Work out the finished part from the listing and answer in its coordinate system (mm). A direction names the side the tool comes from. Coordinates: 2 decimals unless noted, no trailing zeros. Order: outer loops, then holes, each group sorted by start corner. A loop starts at its lowest first (then second) coordinate and runs counter-clockwise, first axis right, second up. Notation, with made-up numbers: M 36.25,84 L 86.25,84 A29 cw 86.25,110 Z; hole C 24.25,37.25 d3. An arc over 180 degrees is marked long. Use a Markdown table: item, result.
from build123d import *

# Parameters (mm, degrees)
ESQUISSE1_R                  = 76.2
ESQUISSE1_R_2                = 60
BOSS_EXTRU_1_DEPTH           = 10
ESQUISSE2_W                  = 30
ESQUISSE2_H                  = 3
BOSS_EXTRU_2_DEPTH           = 480
R_P_TITION_CIRCULAIRE1_COUNT = 4
R_P_TITION_LIN_AIRE1_COUNT   = 2
R_P_TITION_LIN_AIRE1_PITCH   = 490
ESQUISSE5_R                  = 76.2
ESQUISSE5_R_2                = 62.5
BOSS_EXTRU_3_DEPTH           = 10
R_P_TITION_LIN_AIRE2_COUNT   = 2
R_P_TITION_LIN_AIRE2_PITCH   = 170


with BuildPart() as part:
    # Esquisse1 → Boss.-Extru.1 (new body)
    with BuildSketch(Plane(origin=(0, 0, 0), x_dir=(1, 0, 0), z_dir=(0, 1, 0))):
        Circle(ESQUISSE1_R)
        Circle(ESQUISSE1_R_2, mode=Mode.SUBTRACT)
    boss_extru_1 = extrude(amount=BOSS_EXTRU_1_DEPTH)

    # Esquisse2 → Boss.-Extru.2 (add)
    with BuildSketch(Plane(origin=(0, 10, 0), x_dir=(1, 0, 0), z_dir=(0, 1, 0))):
        with Locations((0, 68.920167566)):
            Rectangle(ESQUISSE2_W, ESQUISSE2_H)
    boss_extru_2 = extrude(amount=BOSS_EXTRU_2_DEPTH)

    # Répétition circulaire1: Boss.-Extru.2 ×4 about axis
    r_p_tition_circulaire1_axis = Axis((0, 0, 0), (0, 1, 0))
    for i in range(1, R_P_TITION_CIRCULAIRE1_COUNT):
        add(boss_extru_2.rotate(r_p_tition_circulaire1_axis, i * 360 / R_P_TITION_CIRCULAIRE1_COUNT))

    # Répétition linéaire1: Boss.-Extru.1 ×2
    with Locations(*[(0, i * R_P_TITION_LIN_AIRE1_PITCH, 0) for i in range(1, R_P_TITION_LIN_AIRE1_COUNT)]):
        add(boss_extru_1)

    # Esquisse5 → Boss.-Extru.3 (add)
    with BuildSketch(Plane(origin=(0, 160, 0), x_dir=(1, 0, 0), z_dir=(0, 1, 0))):
        Circle(ESQUISSE5_R)
        Circle(ESQUISSE5_R_2, mode=Mode.SUBTRACT)
    boss_extru_3 = extrude(amount=BOSS_EXTRU_3_DEPTH)

    # Répétition linéaire2: Boss.-Extru.3 ×2
    with Locations(*[(0, i * R_P_TITION_LIN_AIRE2_PITCH, 0) for i in range(1, R_P_TITION_LIN_AIRE2_COUNT)]):
        add(boss_extru_3)


solid = part.part
1. For a pull along Y with two mould halves and no side action, classify faces 6 (the face through (11, 160, 62)), 7 (the face through (-60.47, 164.93, 46.367)), 8 (the face through (0, 414, -67.42)), 9 (the face through (22, 0, 56)) as +Y half, -Y half, draft (parallel to the pull), parting line (faces both ways), or undercut.
Answers below:
| item | result |
|---|---|
| face 6 | undercut |
| face 7 | draft |
| face 8 | undercut |
| face 9 | -Y half |
2. Find the intervals of material crossed by probe 1 along Y at (x, z) = (48.5, -43); probe 2 along X at (y, z) = (334, 0); probe 3 along Z at (x, y) = (0, 2.75), in increasing order.
Answers below:
| item | result |
|---|---|
| probe 1 | 0 to 10, 160 to 170, 330 to 340, 490 to 500 |
| probe 2 | -76.2 to -62.5, 62.5 to 76.2 |
| probe 3 | -76.2 to -60, 60 to 76.2 |
3. Section A-A on y = 212 is taken. Determine the outline of the cut face in (x, z), then the cut area to 3 significant figures.
Answers below:
| item | result |
|---|---|
| outline | M -70.42,-15 L -67.42,-15 L -67.42,15 L -70.42,15 Z; M -15,-70.42 L 15,-70.42 L 15,-67.42 L -15,-67.42 Z; M -15,67.42 L 15,67.42 L 15,70.42 L -15,70.42 Z; M 67.42,-15 L 70.42,-15 L 70.42,15 L 67.42,15 Z |
| area | 360 mm² |
4. For faces 1 (the face through (-67.42, 414, 0)), 2 (the face through (0, 414, -70.42)), 3 (the face through (0, 84, 67.42)), 4 (the face through (0, 414, 70.42)), 5 (the face through (70.42, 84, 0)), determine the directions among +Z, -Z, +X, -X, +Y, -Y from which every point of the face is accessible in a straight line to the end or side of a thin tool.
Answers below:
| item | result |
|---|---|
| face 1 | +Z, -Z |
| face 2 | -Z, +X, -X |
| face 3 | +X, -X |
| face 4 | +Z, +X, -X |
| face 5 | +Z, -Z, +X |
5. Flat-ended cylindrical pins translate along their axes: P1, Ø0.9, axis at y = 217, z = 68.5, coming from the +X side; P2, Ø9, axis at x = 6, y = 90, coming from the -Z side; P3, Ø3.5, axis at y = 428, z = -69, coming from the -X side. Find the tip coordinate at first contact, or state that the pin passes through.
Answers below:
| item | result |
|---|---|
| P1 | x = 15 |
| P2 | z = -70.42 |
| P3 | x = -15 |
6. Section B-B on z = 20.5 is taken. Give the number of separate pieces and of enclosed holes in the cut face, then the cut area to 3 significant figures.
Answers below:
| item | result |
|---|---|
| separate pieces | 8 |
| enclosed holes | 0 |
| area | 1,250 mm² |
